Solid Edge part; units mm, degrees
sketch "Sketch1" plane through (0, 0, 0) normal (0, -1, 0) x (1, 0, 0)
  line L0 (-39.896, 10) -> (30.104, 10)
  line L1 (-39.896, -10) -> (30.104, -10)
  line L2 (-39.896, -10) -> (-39.896, -22.5)
  line L3 (-99.896, -22.5) -> (-39.896, -22.5)
  line L4 (-99.896, -10) -> (-99.896, -22.5)
  line L5 (-99.896, -10) -> (-99.896, -6.077)
  line L6 (-99.896, -6.077) -> (-39.896, 10)
  arc A0 (30.104, 10) -> (30.104, -10) centre (30.104, 0) cw
  circle A1 centre (30.104, 0) radius 5
  circle A2 centre (0, 0) radius 5
  dimension "D1" = 39.896
  dimension "D2" = 39.896
  dimension "D3" = 39.896
  dimension "D4" = 99.896
extrude "Protrusion1" add sketch "Sketch1" along normal mid plane 4
sketch "Sketch2" plane through (-29.896, 0, -6.25) normal (0, -1, 0) x (-0.9659258, 0, -0.258819)
  line L0 (13.0886, 10.2103) -> (16.9709, 24.6992)
  line L1 (16.9709, 24.6992) -> (73.6324, 4.3404)
  line L2 (73.6324, 4.3404) -> (71.0442, -5.3188)
  line L3 (13.0886, 10.2103) -> (71.0442, -5.3188)
extrude "ProtrusiónExtruida_3" add sketch "Sketch2" along normal mid plane 15
sketch "Sketch3" plane through (-69.896, -7.5, -32) normal (-0.9965458, 0, 0.0830455) x (0, -1, 0)
  line L0 (-7.5, 4) -> (-3.5, 0)
  line L1 (-3.5, 0) -> (-11.5, 0)
  line L2 (-7.5, 4) -> (-11.5, 0)
  dimension "D1" = 7.5
  dimension "D2" = 3.5
extrude "Cutout1" cut sketch "Sketch3" along normal through all and the other way through all
properties part number "1976-1500-005" material "Aluminio, 7075-T6"
Geometry check sheet. Reference: the model listing, model coordinates, mm. A direction names the side the tool comes from. Coordinates: 2 decimals unless noted, no trailing zeros. Write each loop counter-clockwise with the first axis right and the second up, starting at its lowest first coordinate (ties: lowest second). Pieces come first, ordered by that corner, then holes. Notation, with made-up numbers: (-7, 6) -> (14, 6) arc R31 cw to (14, 38) -> close; hole circle Ø2 at (84.5, 18.25). An arc over 180 degrees is marked (long way). One line per question, with ' | ' between items.
1. Cross-section at B-B on z = 0. Record the cut outline in (x, y).
Answers:
outline: (-77.22, -2) -> (-5, -2) -> (-5, 2) -> (-77.22, 2) -> close; (5, -2) -> (25.1, -2) -> (25.1, 2) -> (5, 2) -> close; (35.1, -2) -> (40.1, -2) -> (40.1, 2) -> (35.1, 2) -> close
2. Thickness scan on probe 1 along Z at (x, y) = (0, 0.4); probe 2 along Z at (x, y) = (19.5, -0.75); probe 3 along Y at (x, z) = (-60, -9.5). Record the ranges inside material, lowest first. Write a range as from..to.
Answers:
probe 1: z = -10..-5, 5..10 | probe 2: z = -10..10 | probe 3: y = -2..2
3. Cross-section at C-C on x = -47. Record the cut outline in (y, z), and give its area (3 significant figures).
Answers:
outline: (-7.5, -33.91) -> (-4, -33.91) -> (0, -29.89) -> (4, -33.91) -> (7.5, -33.91) -> (7.5, -19.5) -> (2, -19.5) -> (2, 8.1) -> (-2, 8.1) -> (-2, -19.5) -> (-7.5, -19.5) -> close | area: 310 mm²
4. Depth check by flat-ended pin: pin 1 Ø4.5 at (x, y) = (7, 0) entering from -Z; pin 2 Ø16 at (x, z) = (30.104, 0) entering from +Y; pin 3 Ø8 at (x, z) = (-54.5, 4) entering from -Y. Enter the tip coordinate at first touch or a pass-through.
Answers:
pin 1: stops at z = -10 | pin 2: stops at y = 2 | pin 3: stops at y = -2
5. Draft check along X on faces 5 (the flat face through (-69.47, -1.97, -30)), 6 (the flat face through (-29, -2, -5)), 7 (the cylindrical face through (25.11, 0.03, -0.22)). Enter one of: +X half, -X half, draft (parallel to the pull), parting line (faces both ways), or undercut.
Answers:
face 5: -X half | face 6: draft | face 7: undercut
6. Cross-section at A-A on x = 0. Record the cut outline in (y, z).
Answers:
outline: (-2, -10) -> (2, -10) -> (2, -5) -> (-2, -5) -> close; (-2, 5) -> (2, 5) -> (2, 10) -> (-2, 10) -> close
7. Cross-section at D-D on z = -11.5. Record the cut outline in (x, y).
Answers:
outline: (-99.9, -2) -> (-39.9, -2) -> (-39.9, 2) -> (-99.9, 2) -> close
8. Set-up check for faces 1 (the flat face through (-69, 3, -19.5)), 2 (the flat face through (-29, 2, -5)), 3 (the flat face through (-39.896, 0, -27)), 4 (the flat face through (-69.47, 1.97, -30)): record each of +Z, -Z, +X, -X, +Y, -Y from which the full face is reachable in a straight line by a thin tool's end or side.
Answers:
face 1: +Z, +X, -X, +Y | face 2: +Z, +X, -X, +Y | face 3: -Z, +X, +Y, -Y | face 4: -Z, -X
